Can you work these out from the model? Positions are in its coordinate system, mm. A direction names the side the tool comes from. Give positions to 0.01 mm unless a question says otherwise; leave off trailing zeros. Loops run counter-clockwise (first coordinate to the right, second up) from the corner with the lowest first, then second, coordinate; pieces in that order, holes last. Notation, with made-up numbers: (-16, 17.5) -> (2, 17.5) arc R16 ccw to (2, 44.5) -> close; hole circle Ø11 at (29, -17.75). An arc over 180 degrees is marked (long way). Return JSON: item names as keys, results as strings. Group by question number.
Q1. I need wall thicknesses on line 1 along X through (y, z) = (47, 29.5); line 2 along Z through (x, y) = (0, 23); line 3 along Z through (x, y) = (-8.5, 9.5). Which ranges of each line are inside material? Lowest first, please. Write a range as [from, to].
Q2. Suppose I cut it at C-C, the plane x = 0. Please give me the cut outline in (y, z), and give its area (3 significant figures).
Q3. Suppose I cut it at D-D, the plane x = -9. Please give me the cut outline in (y, z).
Q4. Suppose I cut it at B-B, the plane y = -33. Please give me the cut outline in (x, z).
Q5. Suppose I cut it at A-A, the plane z = 31.5. Please give me the cut outline in (x, y).
Q6. Will this pin go through, and if not, where does the flat tip stop? pin 1 (1.5 mm diameter, centred on x = -7, y = 11.5, fed in from +Z).
Q7. Which directions (+Z, -Z, +X, -X, +Y, -Y) give clear straight access to the entire face, cutting with the end or side of a thin tool? Please do faces 1 (the flat face through (34, -1, 34.198)), 2 (the flat face through (23.505, -1, 24)).
Q8. Thinking about a two-plate mould opening in X: for faces 3 (the cylindrical face through (-1.474, 0.889, -6.636)), 4 (the flat face through (-1, -63.5, 11)), 5 (the flat face through (-43.416, -1, 11)), which applies, pulls with the +X half, pulls with the -X half, needs draft (parallel to the pull), parting line crosses it, or undercut?
```python
from build123d import *

# Parameters (mm, degrees)
F0_W     = 19.9103225023
F0_H     = 20.0946768746
F0_R     = 6.7973918103
F1_DEPTH = 63.5


# Not quite as in the source:
# - ends of sketch curves that miss each other by under 0.0002 mm in the source are joined


with BuildPart() as f1:
    # F0 (on Front) → F1 (new body, symmetric)
    with BuildSketch(Plane.XZ):
        with Locations((-33.4604037926, 24.1504837759)):
            Rectangle(F0_W, F0_H)
        Polygon((-23.5052425414, 14.1031453386), (-43.4155650437, 14.1031453386), (-43.4155650437, -13.7344365939), (43.4155575931, -13.7344365939), (43.4155575931, 14.1031453386), (23.5052425414, 14.1031453386), align=None)
        Circle(F0_R, mode=Mode.SUBTRACT)
        Polygon((23.5052425414, 34.1978222132), (23.5052425414, 14.1031453386), (43.4155575931, 14.1031453386), (43.4155650437, 34.1978222132), align=None)
    extrude(amount=F1_DEPTH, both=True)


solid = f1.part
```
Ans:
{
 "1": {"line 1": "x = [-43.42, -23.51], [23.51, 43.42]", "line 2": "z = [-13.73, -6.8], [6.8, 14.1]", "line 3": "z = [-13.73, 14.1]"},
 "2": {"outline": "(-63.5, -13.73) -> (63.5, -13.73) -> (63.5, -6.8) -> (-63.5, -6.8) -> close; (-63.5, 6.8) -> (63.5, 6.8) -> (63.5, 14.1) -> (-63.5, 14.1) -> close", "area": "1,810 mm^2"},
 "3": {"outline": "(-63.5, -13.73) -> (63.5, -13.73) -> (63.5, 14.1) -> (-63.5, 14.1) -> close"},
 "4": {"outline": "(-43.42, -13.73) -> (43.42, -13.73) -> (43.42, 14.1) -> (43.42, 34.2) -> (23.51, 34.2) -> (23.51, 14.1) -> (-23.51, 14.1) -> (-23.51, 34.2) -> (-43.42, 34.2) -> close; hole circle Ø13.59 at (0, 0)"},
 "5": {"outline": "(-43.42, -63.5) -> (-23.51, -63.5) -> (-23.51, 63.5) -> (-43.42, 63.5) -> close; (23.51, -63.5) -> (43.42, -63.5) -> (43.42, 63.5) -> (23.51, 63.5) -> close"},
 "6": {"pin 1": "stops at z = 14.1"},
 "7": {"face 1": "+Z, +X, -X, +Y, -Y", "face 2": "+Z, +Y, -Y"},
 "8": {"face 3": "undercut", "face 4": "needs draft", "face 5": "pulls with the -X half"}
}
